For this review, take the finished solid that the model builds, in its own axes (mm). A direction names the side the tool comes from. Give positions to 0.01 mm unless a question says otherwise; leave off trailing zeros. Write each loop counter-clockwise with the first axis right and the second up, starting at its lowest first coordinate (ties: lowest second). Pieces come first, ordered by that corner, then holes. Notation, with made-up numbers: M 4.25,-40 L 44.25,-40 A16 cw 44.25,-13 Z; hole C 14,9.25 d2. An arc over 180 degrees is marked long. Answer as a JSON object with one key per item and string values. Group by question number.
```python
from build123d import *

# Parameters (mm, degrees)
SKETCH1_R           = 1.75
SKETCH1_R_2         = 3.5
BOSS_EXTRUDE3_DEPTH = 2
SKETCH3_R           = 1.5
BOSS_EXTRUDE4_DEPTH = 12


with BuildPart() as part:
    # Sketch1 → Boss-Extrude3 (new body)
    # profile 1 of 2: a face of its own
    with BuildSketch(Plane(origin=(0, 0, 0), x_dir=(1, 0, 0), z_dir=(0, 1, 0))):
        with BuildLine():
            ThreePointArc((40.05780493, 4.92208645), (19.51761867, 6.504088301), (-0.91087774, 3.843540262))
            ThreePointArc((-0.91087774, 3.843540262), (-3.626704772, -1.56509185), (2.171657179, -3.299455273))
            ThreePointArc((2.171657179, -3.299455273), (19.326940327, 1.634092765), (36.247955143, -4.051229892))
            ThreePointArc((36.247955143, -4.051229892), (38.163769521, -4.895969245), (40.257507506, -4.882165276))
            ThreePointArc((40.257507506, -4.882165276), (45.933967375, -5.003120525), (50.919436714, -7.720089844))
            ThreePointArc((50.919436714, -7.720089844), (50.66068815, -2.80185284), (55.57610439, -2.494136696))
            ThreePointArc((55.57610439, -2.494136696), (48.324550131, 2.276108307), (40.05780493, 4.92208645))
        make_face()
        with Locations(Location((0, 0, 0), (0, 0, 270))):
            Circle(SKETCH1_R, mode=Mode.SUBTRACT)
        with Locations(Location((39.178405, 0, 0), (0, 0, 270))):
            Circle(SKETCH1_R, mode=Mode.SUBTRACT)
    # profile 2 of 2: a face of its own
    with BuildSketch(Plane(origin=(0, 0, 0), x_dir=(1, 0, 0), z_dir=(0, 1, 0))):
        with Locations((53.273794312, -5.13030215)):
            Circle(SKETCH1_R_2)
    extrude(amount=BOSS_EXTRUDE3_DEPTH)

    # Sketch3 → Boss-Extrude4 (add)
    with BuildSketch(Plane(origin=(0, 2, 0), x_dir=(1, 0, 0), z_dir=(0, 1, 0))):
        with Locations(Location((53.273794312, -5.13030215, 0), (0, 0, 270))):
            Circle(SKETCH3_R)
    extrude(amount=BOSS_EXTRUDE4_DEPTH)


solid = part.part
```
Item 1: Insertion check: P1, Ø3, axis at y = 4, z = 3, coming from the -X side; P2, Ø3, axis at x = 39.18, z = 0, coming from the +Y side; P3, Ø3, axis at x = 41, z = -0.5, coming from the +Y side; P4, Ø3, axis at x = 32.5, y = 2.5, coming from the -Z side. Each pin has a flat end and moves straight along its axis. Give the tip position at first contact, or say it passes through.
Item 2: Consider section C-C (z = 6). Give the boundary of the cut face in (x, y), plus the area to 3 significant figures.
Item 3: Machinability: for faces 1 (the cylindrical face through (51.81, 7.92, 4.81)), 2 (the flat face through (33, 0, -1)), which of the approach directions +Z, -Z, +X, -X, +Y, -Y give a long, thin tool a straight path to every point of the face, cutting with its end or side? Answer none if there is none.
Item 4: Draft analysis for pull direction X (two halves, no side actions). For faces 3 (the cylindrical face through (-1.71, 0.99, -0.38)), 4 (the flat face through (26, 2, -1)), 5 (the cylindrical face through (19.81, 0.99, -6.51)), state which applies: released by +X, released by -X, zero draft, split by the parting line, or undercut.
Item 5: To check wall thickness, follow probe 1 along Y at (x, z) = (40, 4); probe 2 along X at (y, z) = (1, 2); probe 3 along Z at (x, y) = (53.5, 7). State the ranges of each line that lie inside material, in increasing order.
Item 6: Consider section B-B (z = 0). Give the boundary of the cut face in (x, y).
Item 7: Consider section D-D (y = 8.5). Give the boundary of the cut face in (x, z), plus the area to 3 significant figures.
Item 8: Consider section A-A (x = 0). Give the boundary of the cut face in (y, z), plus the area to 3 significant figures.
Result set:
{
 "1": {"P1": "stops at x = 51.91", "P2": "passes through", "P3": "stops at y = 2", "P4": "stops at z = -6.14"},
 "2": {"outline": "M 48.47,0 L 56.66,0 L 56.66,2 L 54.5,2 L 54.5,14 L 52.05,14 L 52.05,2 L 48.47,2 Z", "area": "45.7 mm^2"},
 "3": {"face 1": "+Y", "face 2": "+Z, -Z, +X, -X, -Y"},
 "4": {"face 3": "undercut", "face 4": "zero draft", "face 5": "split by the parting line"},
 "5": {"probe 1": "y = 0 to 2", "probe 2": "x = -3.41 to 4.34, 32.99 to 55", "probe 3": "z = 3.65 to 6.61"},
 "6": {"outline": "M -3.95,0 L -1.75,0 L -1.75,2 L -3.95,2 Z; M 1.75,0 L 8.88,0 L 8.88,2 L 1.75,2 Z; M 28.45,0 L 37.43,0 L 37.43,2 L 28.45,2 Z; M 40.93,0 L 52.32,0 L 52.32,2 L 40.93,2 Z"},
 "7": {"outline": "C 53.27,5.13 d3", "area": "7.07 mm^2"},
 "8": {"outline": "M 0,-4.05 L 2,-4.05 L 2,-1.75 L 0,-1.75 Z; M 0,1.75 L 2,1.75 L 2,3.95 L 0,3.95 Z", "area": "9.01 mm^2"}
}
